The figure shows three views and two pictorial views of one solid part (mm, origin at its lowest corner). Answer the questions. A direction names the side the tool comes from. Round coordinates to 2 decimals unless told otherwise and drop trailing zeros. Order: outer loops, then holes, each group sorted by start corner. A loop starts at its lowest first (then second) coordinate and runs counter-clockwise, first axis right, second up. Notation, with made-up numbers: M 17,21 L 64,21 A7 cw 64,25 Z; hole C 6.25,80 d8. An arc over 180 degrees is marked long. Return JSON: item names as keys, results as strings.
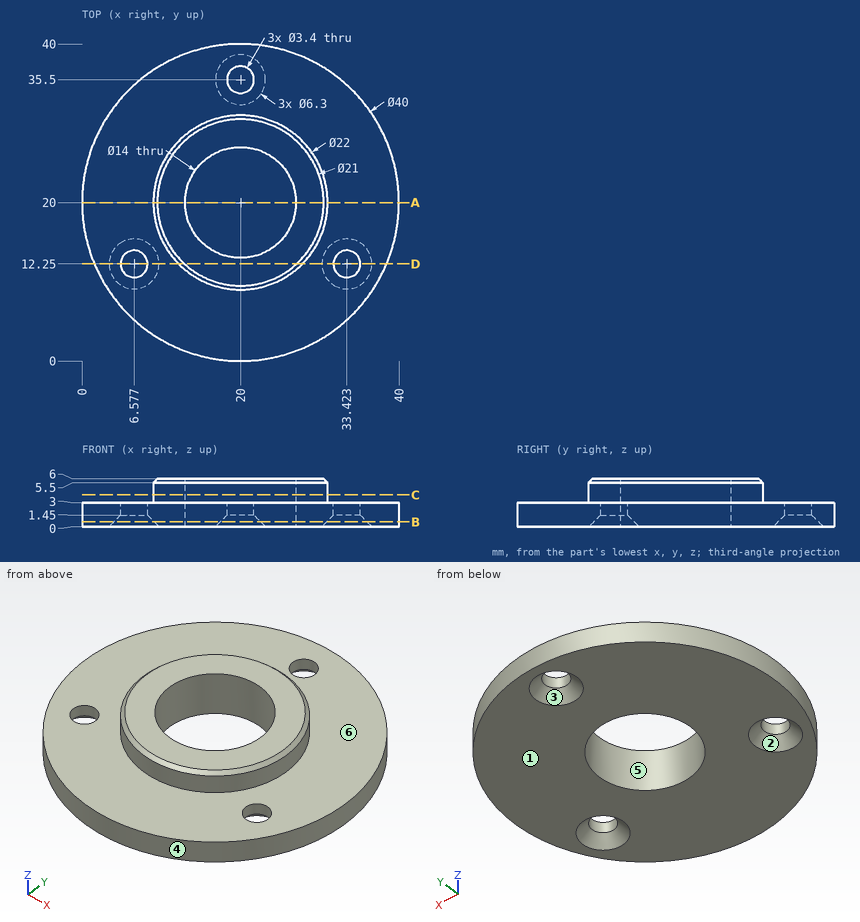
Item 1: Which of the six approach directions +Z, -Z, +X, -X, +Y, -Y give full straight-line access (tool end or side, diameter ignored) to the marked faces 5 and 6?
Output:
{"face 5": "+Z, -Z", "face 6": "+Z"}
Item 2: Each of these flat-tipped pins is pushed along its axis until it touches: pin 1 (1 mm diameter, centred on y = 15.5, z = 3, fed in from -X); pin 2 (5.5 mm diameter, centred on x = 33.42, y = 12.25, fed in from +Z); pin 3 (2 mm diameter, centred on y = 7.5, z = 1.5, fed in from +X). Where does it stop, or does it pass through?
Output:
{"pin 1": "stops at x = 0.4", "pin 2": "stops at z = 3", "pin 3": "stops at x = 36.36"}
Item 3: Find section D-D (y = 12.25). State how many separate pieces and enclosed holes the cut face has.
Output:
{"separate pieces": "3", "enclosed holes": "0"}
Item 4: Consider line 1 along Y through (x, z) = (20.5, 0.6) (1 decimal); line 2 along X through (y, z) = (12.25, 2.35); line 3 along Z through (x, y) = (17.5, 33). Determine where each line is inside the solid, lowest interval first. Write a range as [from, to].
Output:
{"line 1": "y = [0, 13], [27, 33], [38, 40]", "line 2": "x = [1.56, 4.88], [8.28, 31.72], [35.12, 38.44]", "line 3": "z = [0, 3]"}
Item 5: Find section A-A (y = 20). Determine the outline of the cut face in (x, z).
Output:
{"outline": "M 0,0 L 13,0 L 13,6 L 9.5,6 L 9,5.5 L 9,3 L 0,3 Z; M 27,0 L 40,0 L 40,3 L 31,3 L 31,5.5 L 30.5,6 L 27,6 Z"}
Item 6: Find section C-C (z = 4). Determine the outline of the cut face in (x, y).
Output:
{"outline": "C 20,20 d22; hole C 20,20 d14"}
Item 7: Find section B-B (z = 0.6). Determine the outline of the cut face in (x, y), plus the area to 3 significant figures.
Output:
{"outline": "C 20,20 d40; hole C 6.58,12.25 d5.1; hole C 20,20 d14; hole C 20,35.5 d5.1; hole C 33.42,12.25 d5.1", "area": "1,040 mm^2"}
Item 8: The mould has two halves that part along X. Classify the marked faces 1, 2, 3 and 4: pulls with the +X half, pulls with the -X half, needs draft (parallel to the pull), parting line crosses it, or undercut.
Output:
{"face 1": "needs draft", "face 2": "undercut", "face 3": "undercut", "face 4": "parting line crosses it"}
